Read the model definition and answer for the solid it produces. Units are mm, in the model's axes. A direction names the side the tool comes from. Round coordinates to 2 decimals unless told otherwise and drop trailing zeros. Loops run counter-clockwise (first coordinate to the right, second up) from the corner with the lowest first, then second, coordinate; pieces in that order, holes last. Notation, with made-up numbers: (42.5, -36) -> (87.5, -36) arc R16 ccw to (87.5, -27) -> close; hole circle Ø9 at (14.25, 64.25). An arc over 180 degrees is marked (long way). Put each result on its own line as item: value.
Autodesk Inventor part; units mm, degrees
ref_plane "YZ Plane" through (0, 0, 0) normal (1, 0, 0) x (0, 1, 0)
ref_plane "XZ Plane" through (0, 0, 0) normal (0, 1, 0) x (-1, 0, 0)
ref_plane "XY Plane" through (0, 0, 0) normal (0, 0, 1) x (1, 0, 0)
sketch "スケッチ3" plane through (0, 0, 0) normal (0, 0, 1) x (1, 0, 0)
  circle A0 centre (0, 0) radius 1.5
  circle A1 centre (0, 0) radius 3
  line L0 (3, 0) -> (3, -4)
  line L1 (3, -4) -> (-3, -4)
  line L2 (-3, -4) -> (-3, 0)
  dimension "d9" = 6
  dimension "d8" = 3
  dimension "d10" = 4
extrude "押し出し3" add sketch "スケッチ3" along normal blind 4
sketch "スケッチ4" plane through (-3, -4, 0) normal (0, -1, 0) x (1, 0, 0)
  line L0 (6, 4) -> (0, 4)
  line L1 (6, 0) -> (6, 4)
  circle A0 centre (3, 2) radius 3
  line L2 (0, 0) -> (0, 4)
  line L3 (4.0287, 2) -> (1.8756, 2)
  point P0 (3, 0)
  point P1 (6, 2)
extrude "押し出し4" cut sketch "スケッチ4" against normal blind 10 contours A0 L0 | L0 A0 keep common part
extrude "押し出し5" add sketch "スケッチ4" along normal blind 4 contours A0 L0 | L0 A0
properties part number "頭" material "ABS プラスチック"
Item 1: The part is cut by section B-B (z = 2.3). Determine the outline of the cut face in (x, y).
Derived:
outline: (-2.98, -8) -> (2.98, -8) -> (2.98, 0.3) arc R3 ccw to (-2.98, 0.3) -> close; hole circle Ø3 at (0, 0)
Item 2: The part is cut by section A-A (x = 0). Determine the outline of the cut face in (y, z), then the cut area to 3 significant figures.
Derived:
outline: (-8, -1) -> (-4, -1) -> (-4, 0) -> (-1.5, 0) -> (-1.5, 4) -> (-4, 4) -> (-4, 5) -> (-8, 5) -> close; (1.5, 0) -> (3, 0) -> (3, 4) -> (1.5, 4) -> close
area: 40.0 mm^2
Item 3: Find the intervals of material crossed by line 1 along Y through (x, z) = (0, 1.6); line 2 along Y through (x, z) = (1.3, 4.2); line 3 along Z through (x, y) = (2.15, 1), in increasing order.
Derived:
line 1: y = -8 to -1.5, 1.5 to 3
line 2: y = -8 to -4
line 3: z = 0 to 4
Item 4: For a pull along Y with two mould halves and no side action, classify faces 1 (the flat face through (0, -2, 4)), 2 (the flat face through (0, -8, 2)), 3 (the cylindrical face through (-1.5, -0.07, 1.97)), 4 (the cylindrical face through (0, 3, 2)) as pulls with the +Y half, pulls with the -Y half, needs draft (parallel to the pull), parting line crosses it, or undercut.
Derived:
face 1: needs draft
face 2: pulls with the -Y half
face 3: undercut
face 4: pulls with the +Y half
Item 5: Which of the six approach directions +Z, -Z, +X, -X, +Y, -Y give full straight-line access (tool end or side, diameter ignored) to faces 5 (the flat face through (0, -4, 4.4)), 6 (the cylindrical face through (2.775, -4.181, 3.141)), 7 (the flat face through (0, -4, -0.4))?
Derived:
face 5: +Z, +X, -X, +Y
face 6: +Y, -Y
face 7: -Z, +X, -X, +Y
Item 6: The part is cut by section C-C (y = -1.25). Determine the outline of the cut face in (x, z).
Derived:
outline: (-2.24, 0) -> (-0.83, 0) -> (-0.83, 4) -> (-2.24, 4) arc R3 ccw to start; (0.83, 0) -> (2.24, 0) arc R3 ccw to (2.24, 4) -> (0.83, 4) -> close
Item 7: The part is cut by section D-D (x = -0.75). Determine the outline of the cut face in (y, z), then the cut area to 3 significant figures.
Derived:
outline: (-8, -0.9) -> (-4, -0.9) -> (-4, 0) -> (-1.3, 0) -> (-1.3, 4) -> (-4, 4) -> (-4, 4.9) -> (-8, 4.9) -> close; (1.3, 0) -> (2.9, 0) -> (2.9, 4) -> (1.3, 4) -> close
area: 40.5 mm^2
Item 8: Flat-ended cylindrical pins translate along their axes: pin 1 Ø1.3 at (x, y) = (1, 0.5) entering from +Z; pin 2 Ø1.3 at (x, y) = (0.5, 0) entering from -Z; pin 3 Ø2 at (x, y) = (2.5, -4.5) entering from +Z; pin 4 Ø1.5 at (y, z) = (-2, 1) entering from +X. Find the tip coordinate at first contact, or state that the pin passes through.
Derived:
pin 1: stops at z = 4
pin 2: passes through
pin 3: stops at z = 4.6
pin 4: stops at x = 2.99
